```python
from build123d import *

# Parameters (mm, degrees)
BOSS_EXTRUDE1_DEPTH = 23


with BuildPart() as part:
    # Sketch1 → Boss-Extrude1 (new body)
    with BuildSketch(Plane(origin=(0, 0, 0), x_dir=(1, 0, 0), z_dir=(0, 1, 0))):
        Polygon((5.366336563, 43.198240053), (8.849047037, 44.93959529), (35.152676147, 49.613759348), (35.152676147, 53.829672027), (47.067211981, 53.829672027), (48.991867769, 57.862284156), (55.040785962, 57.862284156), (56.96544175, 53.829672027), (68.879977584, 53.829672027), (68.879977584, 49.613759348), (95.183606694, 44.93959529), (98.666317168, 43.198240053), (98.666317168, 22.668578308), (93.808852559, 22.668578308), (91.808852559, 22.668578308), (91.808852559, 26.884490988), (81.252764796, 26.884490988), (81.252764796, 21.110523622), (74.65394495, 21.110523622), (74.65394495, 25.876337956), (64.022512975, 25.876337956), (64.022512975, 3.422020423), (57.31833656, -3.282155992), (46.714317171, -3.282155992), (40.010140756, 3.422020423), (40.010140756, 25.876337956), (29.378708781, 25.876337956), (29.378708781, 21.110523622), (22.779888935, 21.110523622), (22.779888935, 26.884490988), (12.223801172, 26.884490988), (12.223801172, 22.668578308), (10.223801172, 22.668578308), (5.366336563, 22.668578308), align=None)
    extrude(amount=BOSS_EXTRUDE1_DEPTH)


solid = part.part
```
Read the model definition and answer for the solid it produces. Units are mm, in the model's axes. A direction names the side the tool comes from. Give positions to 0.01 mm unless a question says otherwise; leave off trailing zeros. Order: outer loops, then holes, each group sorted by start corner. A loop starts at its lowest first (then second) coordinate and runs counter-clockwise, first axis right, second up.
(1) For faces 1 (the flat face through (41, 11, -53.83)), 2 (the flat face through (9, 11, -22.669)), 3 (the flat face through (60.7, 11.3, -0.1)), 4 (the flat face through (87, 11, -26.884)), 5 (the flat face through (68.88, 11, -52)), determine the directions among +Z, -Z, +X, -X, +Y, -Y from which every point of the face is accessible in a straight line to the end or side of a thin tool.
(2) Straight lines are drawn through the part: L1, parallel to X at y = 9, z = -23.5; L2, parallel to X at y = 13.5, z = -26; L3, parallel to X at y = 10.25, z = -6. For each, find the intervals that lie inside material, in ascending order.
(3) Given pin 1 (5 mm diameter, centred on x = 37, y = 8, fed in from -Z); pin 2 (2 mm diameter, centred on y = 11, z = -52, fed in from -X); pin 3 (5.5 mm diameter, centred on x = 86.5, y = 8, fed in from +Z); pin 4 (10 mm diameter, centred on x = 24.5, z = -14, fed in from +Y), each flat-ended and moving along its own axis, determine where each tip first touches the part or whether it passes through.
(4) Find section B-B (x = 36.5). Give the vertices of the cut face in (y, z).
(5) Find section C-C (z = -10.5). Give the vertices of the cut face in (x, y).
Result sheet:
1. face 1: -Z, -X, +Y, -Y
1. face 2: +Z, -X, +Y, -Y
1. face 3: +Z, +X, +Y, -Y
1. face 4: +Z, +Y, -Y
1. face 5: -Z, +X, +Y, -Y
2. L1: x = 5.37 to 12.22, 22.78 to 29.38, 40.01 to 64.02, 74.65 to 81.25, 91.81 to 98.67
2. L2: x = 5.37 to 12.22, 22.78 to 81.25, 91.81 to 98.67
2. L3: x = 40.01 to 64.02
3. pin 1: stops at z = -53.83
3. pin 2: stops at x = 35.15
3. pin 3: stops at z = -26.88
3. pin 4: passes through
4. outline: (0, -53.83) - (23, -53.83) - (23, -25.88) - (0, -25.88) - close
5. outline: (40.01, 0) - (64.02, 0) - (64.02, 23) - (40.01, 23) - close
